Build history of the part. All positions in model axes, mm. A direction names the side the tool comes from. Round coordinates to 2 decimals unless told otherwise and drop trailing zeros. One line per question, with ' | ' between items.
from build123d import *

# Parameters (mm, degrees)
BOSS_EXTRUDE1_DEPTH = 20
SKETCH2_W           = 80
SKETCH2_H           = 60
CUT_EXTRUDE1_DEPTH  = 20
CUT_EXTRUDE2_DEPTH  = 20
SKETCH5_R           = 1
CUT_EXTRUDE4_DEPTH  = 1


with BuildPart() as part:
    # Sketch1 → Boss-Extrude1 (new body)
    with BuildSketch(Plane.XY):
        with BuildLine():
            Line((0, 55), (47.027150271, 55))
            ThreePointArc((47.027150271, 55), (54.098218083, 52.071067812), (57.027150271, 45))
            Line((57.027150271, 45), (57.027150271, -45))
            ThreePointArc((57.027150271, -45), (54.098218083, -52.071067812), (47.027150271, -55))
            Line((47.027150271, -55), (0.441720212, -55))
            ThreePointArc((0.441720212, -55), (-0.005784399, -54.989981963), (-0.452392388, -54.959947924))
            add(Edge.make_bspline(
                [(-81.211824921, 0), (-80.030487626, -16.829502098), (-64.338425338, -33.147030622), (-38.651767748, -47.067005008), (-19.235585963, -52.655551102), (-6.275521273, -54.437200923), (-0.452392388, -54.959947924)],
                knots=[0, 0, 0, 0, 0.422832961, 0.624311743, 0.828189209, 0.995662594, 0.995662594, 0.995662594, 0.995662594], degree=3))
            add(Edge.make_bspline(
                [(-81.211824921, 0), (-80.03021452, 16.829535827), (-64.338739167, 33.146991864), (-33.323213758, 49.95438824), (-13.059438762, 53.859901845), (0, 55)],
                knots=[0, 0, 0, 0, 0.422843906, 0.624327904, 1, 1, 1, 1], degree=3))
        make_face()
    extrude(amount=BOSS_EXTRUDE1_DEPTH)

    # Sketch2 → Cut-Extrude1 (cut)
    with BuildSketch(Plane.XY.offset(20)):
        with Locations((-7.289359696, 0)):
            Rectangle(SKETCH2_W, SKETCH2_H)
    extrude(amount=-CUT_EXTRUDE1_DEPTH, mode=Mode.SUBTRACT)

    # Sketch3 → Cut-Extrude2 (cut)
    with BuildSketch(Plane.XY.offset(20)):
        Polygon((57.027150271, 6.8), (49.227150271, 6.8), (49.227150271, 2.5), (44.527150271, 2.5), (44.527150271, 0), (49.227150271, 0), (49.227150271, -15.9), (57.027150271, -15.9), align=None)
    extrude(amount=-CUT_EXTRUDE2_DEPTH, mode=Mode.SUBTRACT)

    # Sketch5 → Cut-Extrude4 (cut)
    with BuildSketch(Plane.XZ.offset(-2.5)):
        with Locations((46.927150271, 10)):
            Circle(SKETCH5_R)
    extrude(amount=-CUT_EXTRUDE4_DEPTH, mode=Mode.SUBTRACT)


solid = part.part
Q1. Drop flat-ended pins along their axis: pin 1 (8.5 mm diameter, centred on x = 51.5, z = 8.5, fed in from -Y); pin 2 (5 mm diameter, centred on y = -11.5, z = 13.5, fed in from +X); pin 3 (6 mm diameter, centred on x = 54.5, z = 13, fed in from +Y). Give the stop position or say it passes through.
Found:
pin 1: y = -55 | pin 2: x = 49.23 | pin 3: y = 53.94
Q2. Which spindle directions (+Z, -Z, +X, -X, +Y, -Y) get a long thin tool onto all of the face, cutting with end or side? Do faces 5 (the flat face through (32.711, 0, 10)), 6 (the flat face through (49.227, 5, 10)), 7 (the flat face through (23, 55, 10)). Say none if no direction does.
Found:
face 5: +Z, -Z | face 6: +Z, -Z, +X | face 7: +Z, -Z, +X, -X, +Y
Q3. Drill centre lines: L1, parallel to Y at x = 0, z = 12; L2, parallel to Y at x = 45, z = 15; L3, parallel to X at y = -11.5, z = 18.5. Where is each one in solid material? Low to high. Write a range as from..to.
Found:
L1: -54.99..-30, 30..55 | L2: -55..0, 2.5..55 | L3: -78.71..-47.29, 32.71..49.23
Q4. Pull direction X, two halves, no side cores. Call faces 1 (the flat face through (-8, -30, 10)), 2 (the flat face through (35, 1, 0)), 3 (the flat face through (-47.289, 0, 10)), 4 (the flat face through (57.027, -30, 10)): +X half, -X half, draft (parallel to the pull), parting line (faces both ways), or undercut.
Found:
face 1: undercut | face 2: draft | face 3: undercut | face 4: +X half
